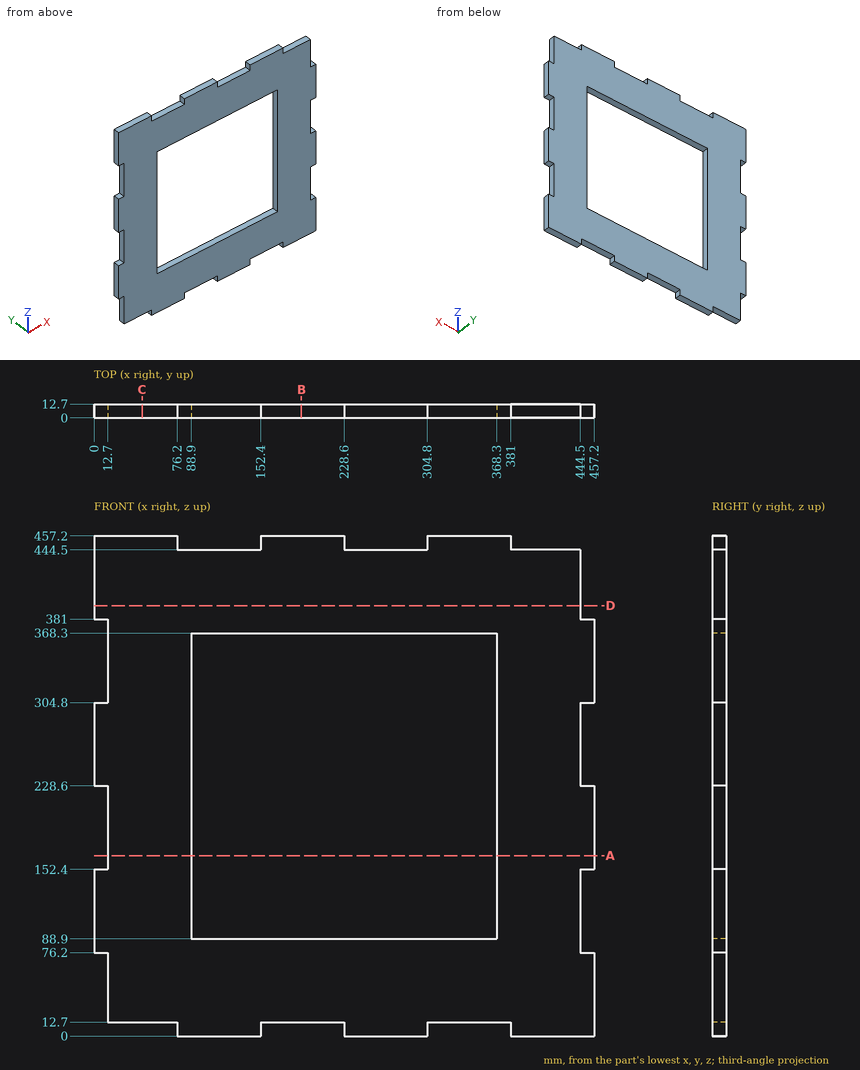
Print and shaded views of the part. All mm, measured from the part's lowest x, y and z. Give positions to 0.01 mm unless a question says otherwise; leave off trailing zeros. Order: outer loops, then holes, each group sorted by start corner. A loop starts at its lowest first (then second) coordinate and runs counter-clockwise, first axis right, second up. Notation, with made-up numbers: (-35, 74.5) - (-17, 74.5) arc R26 cw to (-17, 101.5) - close; hole circle Ø6 at (-7.5, 46.5). An arc over 180 degrees is marked (long way). Use a Markdown table: item, result.
1) Flat gauge pins, fed straight in: P1, Ø4, axis at y = 5.5, z = 401.5, coming from the +X side; P2, Ø6.5, axis at x = 451.5, y = 7.5, coming from the +Z side; P3, Ø6.5, axis at x = 412, y = 8.5, coming from the +Z side; P4, Ø6, axis at y = 7, z = 77.5, coming from the -X side. Where does each tip first touch, or does it go through?
Checked values:
| item | result |
|---|---|
| P1 | x = 444.5 |
| P2 | z = 381 |
| P3 | z = 444.5 |
| P4 | x = 0 |
2) Saw through at B-B on x = 189.5. List the corners of the cut face in (y, z).
Checked values:
| item | result |
|---|---|
| outline | (0, 12.7) - (12.7, 12.7) - (12.7, 88.9) - (0, 88.9) - close; (0, 368.3) - (12.7, 368.3) - (12.7, 457.2) - (0, 457.2) - close |
3) Saw through at C-C on x = 44. List the corners of the cut face in (y, z).
Checked values:
| item | result |
|---|---|
| outline | (0, 12.7) - (12.7, 12.7) - (12.7, 457.2) - (0, 457.2) - close |
4) Saw through at D-D on z = 393.5. List the corners of the cut face in (x, y), plus the area to 3 significant figures.
Checked values:
| item | result |
|---|---|
| outline | (0, 0) - (444.5, 0) - (444.5, 12.7) - (0, 12.7) - close |
| area | 5,650 mm² |
5) Saw through at A-A on z = 165. List the corners of the cut face in (x, y).
Checked values:
| item | result |
|---|---|
| outline | (12.7, 0) - (88.9, 0) - (88.9, 12.7) - (12.7, 12.7) - close; (368.3, 0) - (457.2, 0) - (457.2, 12.7) - (368.3, 12.7) - close |
6) Probe L1, parallel to X at y = 2, z = 258.5; L2, parallel to X at y = 4.25, z = 187. List the from-to ranges inside material, lowest first. Write a range as from..to.
Checked values:
| item | result |
|---|---|
| L1 | 0..88.9, 368.3..444.5 |
| L2 | 12.7..88.9, 368.3..457.2 |
